Could you check a few things on this model? Use its own coordinates, in mm. Face numbers are marked on the shaded views. A direction names the side the tool comes from. Coordinates: 2 decimals unless noted, no trailing zeros. Loops run counter-clockwise (first coordinate to the right, second up) from the corner with the lowest first, then second, coordinate; pieces in that order, holes last. Notation, with made-up numbers: (-38.75, 48) - (20.25, 48) arc R18 cw to (20.25, 52) - close; hole circle Ø4 at (61.5, 56.5). An arc over 180 degrees is marked (long way). One line per item, written item: value. Start each with the question number.
(1) If we section it at C-C on y = 1.75: Write out the boundary of the cut face in (x, z).
(2) If we section it at D-D on y = -6.25: Write out the boundary of the cut face in (x, z), then the cut area to 3 significant figures.
(3) If we section it at B-B on x = 5: Write out the boundary of the cut face in (y, z).
(4) If we section it at A-A on z = 2.55: Write out the boundary of the cut face in (x, y), then the cut area to 3 significant figures.
(5) On a 3-axis mill with a long thin cutter (end or side, diameter ignored), from which of +Z, -Z, +X, -X, +Y, -Y can I reach the whole of each face in a straight line? I mean the marked faces 1, 2 and 3. Say none if no direction works.
(6) I'm going to push flat-ended pins straight in: P1, Ø3, axis at x = -3.5, y = 3, coming from the -Z side; P2, Ø1, axis at y = -1, z = 1.5, coming from the +X side; P3, Ø1.5, axis at x = 5.5, y = -2.5, coming from the -Z side; P4, Ø1, axis at x = 6.5, z = 1, coming from the -Y side. Where does each tip first touch, or does it pass through?
(7) If I drill on line 1 along X through (y, z) = (-3, 1.95); line 2 along Z through (x, y) = (-4, 3.5); line 3 along Y through (x, z) = (1.25, 0.65), over which ranges is the centre line in solid material (lowest first)? Write a range as from..to.
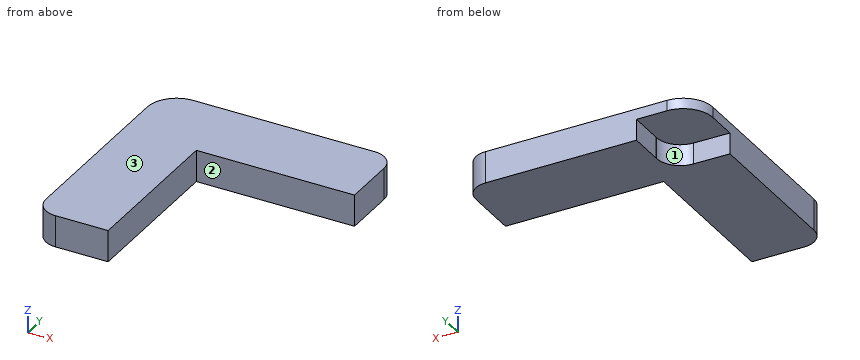
```python
from build123d import *

# Parameters (mm, degrees)
F1_DEPTH = 3
F2_R     = 2.8
F3_R     = 2
F5_DEPTH = 2


with BuildPart() as f1:
    # F0 (on Top) → F1 (new body)
    with BuildSketch(Plane.XY):
        Polygon((0, -15), (0, 0), (15, 0), (15, 7), (-7, 7), (-7, -15), align=None)
    extrude(amount=F1_DEPTH)

    # F2
    f2_edges = [f1.edges().sort_by_distance(p)[0] for p in [
        (-7, 7, 1.5),
    ]]
    fillet(f2_edges, radius=F2_R)

    # F3
    f3_edges = [f1.edges().sort_by_distance(p)[0] for p in [
        (15, 7, 1.5),
        (-7, -15, 1.5),
    ]]
    fillet(f3_edges, radius=F3_R)

    # F4 (on face) → F5 (cut)
    with BuildSketch(Plane(origin=(0, 0, 0), x_dir=(1, 0, 0), z_dir=(0, 0, -1))):
        with BuildLine():
            ThreePointArc((-1.322323, -3.644969), (-1.321403, -3.60783), (-1.321097, -3.570682))
            ThreePointArc((-1.321097, -3.570682), (-1.971123, -1.988726), (-3.545615, -1.320826))
            ThreePointArc((-3.545615, -1.320826), (-5.196971, -5.126005), (-1.322323, -3.644969))
        make_face()
        with BuildLine():
            ThreePointArc((-1.322323, -3.644969), (-5.196971, -5.126005), (-3.545615, -1.320826))
            Line((-3.545615, -1.320826), (-7, -1.281702))
            Line((-7, -1.281702), (-7, -4.2))
            ThreePointArc((-7, -4.2), (-6.179899, -6.179899), (-4.2, -7))
            Line((-4.2, -7), (-1.322323, -7))
            Line((-1.322323, -7), (-1.322323, -3.644969))
        make_face()
    extrude(amount=-F5_DEPTH, mode=Mode.SUBTRACT)


solid = f1.part
```
Values:
1. outline: (-7, 2) - (-2.25, 2) - (-2.25, 0) - (15, 0) - (15, 3) - (-7, 3) - close
2. outline: (-7, 0) - (0, 0) - (0, 3) - (-7, 3) - close
2. area: 21.0 mm2
3. outline: (0, 0) - (7, 0) - (7, 3) - (0, 3) - close
4. outline: (-7, -13) arc R2 ccw to (-5, -15) - (0, -15) - (0, 0) - (15, 0) - (15, 5) arc R2 ccw to (13, 7) - (-4.2, 7) arc R2.8 ccw to (-7, 4.2) - close
4. area: 256 mm2
5. face 1: -Z, -X, +Y
5. face 2: +Z, -Z, +X, -Y
5. face 3: +Z, +X, -X, +Y, -Y
6. P1: stops at z = 2
6. P2: stops at x = 0
6. P3: passes through
6. P4: stops at y = 0
7. line 1: x = -7..0
7. line 2: z = 2..3
7. line 3: y = 0..7
